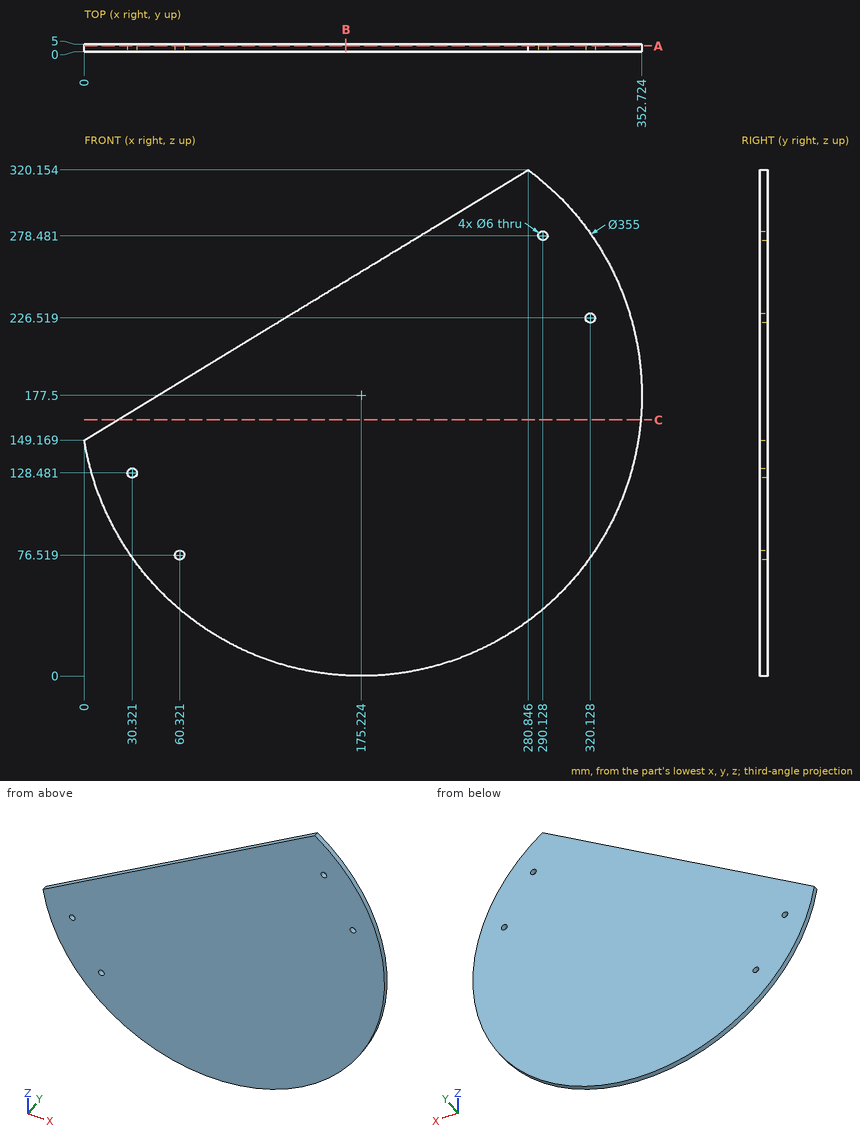
Here's the drawing with two shaded views (mm, measured from the low corner). I have some questions. Round coordinates to 2 decimals unless told otherwise and drop trailing zeros. Loops run counter-clockwise (first coordinate to the right, second up) from the corner with the lowest first, then second, coordinate; pieces in that order, holes last.
1. Suppose I cut it at C-C, the plane z = 162. Please give me the cut outline in (x, y) (1 decimal).
Answers:
outline: (21.1, 0) - (352, 0) - (352, 5) - (21.1, 5) - close
2. Will these pins go through, and if not, where does the flat tip stop? pin 1 (1 mm diameter, centred on x = 74, y = 3, fed in from +Z) (1 decimal); pin 2 (1.5 mm diameter, centred on y = 3.5, z = 159, fed in from -X) (1 decimal).
Answers:
pin 1: stops at z = 194.5
pin 2: stops at x = 14.9
3. Suppose I cut it at B-B, the plane x = 165.5. Please give me the cut outline in (y, z), and give its area (3 significant figures).
Answers:
outline: (0, 0.27) - (5, 0.27) - (5, 249.93) - (0, 249.93) - close
area: 1,250 mm2
4. If I drill on probe 1 along X at (y, z) = (4.4, 126) (1 decimal); probe 2 along X at (y, z) = (1, 226.5) (1 decimal); probe 3 along X at (y, z) = (2.15, 140.5) (1 decimal), over which ranges is the centre line in solid material (lowest first)?
Answers:
probe 1: x = 5.4 to 28.6, 32 to 345.1
probe 2: x = 127 to 317.1, 323.1 to 345.8
probe 3: x = 1.6 to 348.8
5. Suppose I cut it at A-A, the plane y = 3.8. Please give me the cut outline in (x, z) (1 decimal).
Answers:
outline: (0, 149.2) arc R177.5 ccw (long way) to (280.8, 320.2) - close; hole circle Ø6 at (30.3, 128.5); hole circle Ø6 at (60.3, 76.5); hole circle Ø6 at (290.1, 278.5); hole circle Ø6 at (320.1, 226.5)
